Answer from the drawing. Dimensions are ordinates in mm from the lowest x, y and z of the part. A direction names the side the tool comes from. Round coordinates to 2 decimals unless told otherwise and drop trailing zeros. Loops run counter-clockwise (first coordinate to the right, second up) from the corner with the lowest first, then second, coordinate; pieces in that order, holes last. Notation, with made-up numbers: (47, 52.25) - (81, 52.25) arc R18 cw to (81, 66.25) - close; hole circle Ø2 at (-20, 82). An arc over 180 degrees is marked (long way). Answer as CSV lines item,"result".
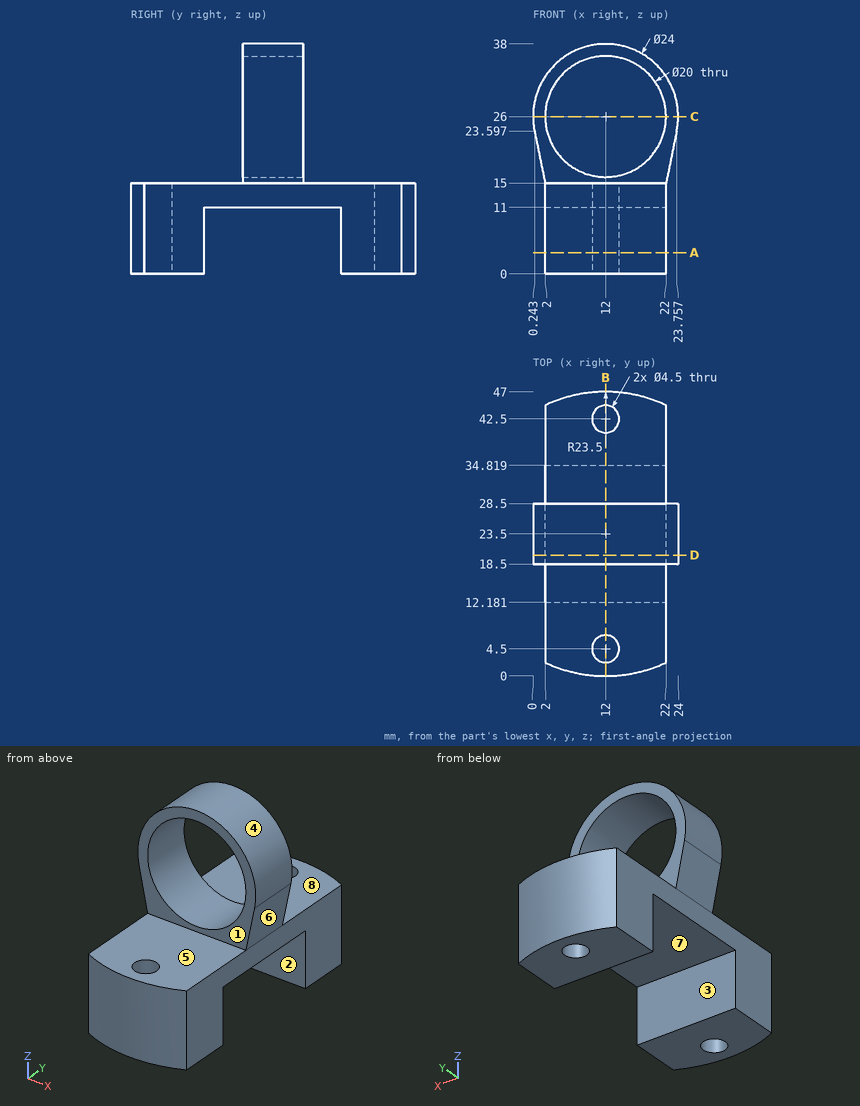
1) A cutting plane is placed at B-B, the plane x = 12. Determine the outline of the cut face in (y, z).
Entries:
outline,"(0, 0) - (2.25, 0) - (2.25, 15) - (0, 15) - close; (6.75, 0) - (12.18, 0) - (12.18, 11) - (34.82, 11) - (34.82, 0) - (40.25, 0) - (40.25, 15) - (28.5, 15) - (28.5, 16) - (18.5, 16) - (18.5, 15) - (6.75, 15) - close; (18.5, 36) - (28.5, 36) - (28.5, 38) - (18.5, 38) - close; (44.75, 0) - (47, 0) - (47, 15) - (44.75, 15) - close"
2) The mould has two halves that part along Y. Classify the marked faces 1, 2, 3 and 4: pulls with the +Y half, pulls with the -Y half, needs draft (parallel to the pull), parting line crosses it, or undercut.
Entries:
face 1,"pulls with the -Y half"
face 2,"undercut"
face 3,"undercut"
face 4,"needs draft"
3) Find the intervals of material crossed by line 1 (Y direction, x = 12, z = 5.25); line 2 (Y direction, x = 12, z = 11.25); line 3 (Z direction, x = 12, y = 24.75), in increasing order.
Entries:
line 1,"y = 0 to 2.25, 6.75 to 12.18, 34.82 to 40.25, 44.75 to 47"
line 2,"y = 0 to 2.25, 6.75 to 40.25, 44.75 to 47"
line 3,"z = 11 to 16, 36 to 38"
4) A tool of negligible diameter and unlimited length cuts with its end or side. For the marked faces 5, 6, 7 and 8, from which of +Z, -Z, +X, -X, +Y, -Y can it reach the whole face along a straight path? Write none if from no direction.
Entries:
face 5,"+Z, +X, -X, -Y"
face 6,"-Z, +X, +Y, -Y"
face 7,"-Z, +X, -X"
face 8,"+Z, +X, -X, +Y"
5) A cutting plane is placed at D-D, the plane y = 20. Determine the outline of the cut face in (x, z), plus the area to 3 significant figures.
Entries:
outline,"(0.24, 23.6) - (2, 15) - (2, 11) - (22, 11) - (22, 15) - (23.76, 23.6) arc R12 ccw (long way) to start; hole circle Ø20 at (12, 26)"
area,"236 mm^2"
6) A cutting plane is placed at A-A, the plane z = 3.5. Determine the outline of the cut face in (x, y).
Entries:
outline,"(2, 2.23) arc R23.5 ccw to (22, 2.23) - (22, 12.18) - (2, 12.18) - close; (2, 34.82) - (22, 34.82) - (22, 44.77) arc R23.5 ccw to (2, 44.77) - close; hole circle Ø4.5 at (12, 4.5); hole circle Ø4.5 at (12, 42.5)"
7) A cutting plane is placed at C-C, the plane z = 26. Determine the outline of the cut face in (x, y).
Entries:
outline,"(0, 18.5) - (2, 18.5) - (2, 28.5) - (0, 28.5) - close; (22, 18.5) - (24, 18.5) - (24, 28.5) - (22, 28.5) - close"
8) Each of these flat-tipped pins is pushed along its axis until it touches: P1, Ø7, axis at x = 12, y = 42.5, coming from the +Z side; P2, Ø12, axis at y = 12, z = 19.5, coming from the +X side; P3, Ø1.5, axis at x = 16.5, z = 4, coming from the +Y side. Where does it stop, or does it pass through?
Entries:
P1,"stops at z = 15"
P2,"stops at x = 22"
P3,"stops at y = 46.7"
